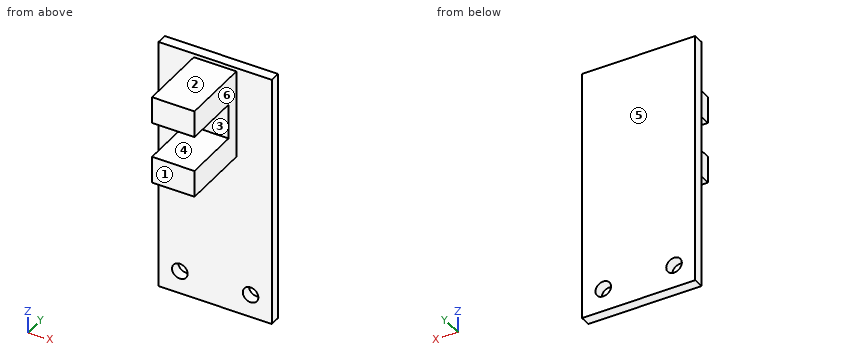
```python
from build123d import *

# Parameters (mm, degrees)
F0_W     = 16
F0_H     = 36
F0_R     = 1.1
F1_DEPTH = 1.47957
F3_W     = 6
F3_H     = 3.8
F4_DEPTH = 10
F3_H_2   = 4.992
F5_DEPTH = 1.85


with BuildPart() as f1:
    # F0 (on Front) → F1 (new body)
    with BuildSketch(Plane.XZ):
        with Locations((8, -18)):
            Rectangle(F0_W, F0_H)
        with Locations((3, -32.75)):
            Circle(F0_R, mode=Mode.SUBTRACT)
        with Locations((13, -32.75)):
            Circle(F0_R, mode=Mode.SUBTRACT)
    extrude(amount=F1_DEPTH)

    # F3 (on face) → F4 (join)
    with BuildSketch(Plane.XZ.offset(1.47957)):
        with Locations((8, -11.192)):
            Rectangle(F3_W, F3_H)
        with Locations((8, -2.4)):
            Rectangle(F3_W, F3_H)
    extrude(amount=F4_DEPTH)

    # F3 (on face) → F5 (join)
    with BuildSketch(Plane.XZ.offset(1.47957)):
        with Locations((8, -6.796)):
            Rectangle(F3_W, F3_H_2)
    extrude(amount=F5_DEPTH)


solid = f1.part
```
Check sheet for the modelled part. Datum: model origin and axes. Units: mm. Face numbers are marked on the shaded views. A direction names the side the tool comes from. Give positions to 0.01 mm unless a question says otherwise; leave off trailing zeros. Order: outer loops, then holes, each group sorted by start corner. A loop starts at its lowest first (then second) coordinate and runs counter-clockwise, first axis right, second up. Notation, with made-up numbers: M 58.25,-4.5 L 87.25,-4.5 A23 ccw 87.25,33.5 Z; hole C 65.25,62.25 d11. An arc over 180 degrees is marked long. Answer in a Markdown table with one row per item. Add a question column.
Q1. Thickness scan on L1, parallel to Z at x = 3, y = -0.55; L2, parallel to Z at x = 10.75, y = -10.5; L3, parallel to Y at x = 9, z = -5. Record the ranges inside material, lowest first.
Q2. Sectioned sample at C-C, the plane z = -32.75. Record the boundary of the cut face in (x, y), and give its area (3 significant figures).
Q3. Sectioned sample at A-A, the plane x = 13. Record the boundary of the cut face in (y, z), and give its area (3 significant figures).
Q4. Sectioned sample at D-D, the plane x = 7. Record the boundary of the cut face in (y, z), and give its area (4 significant figures).
Q5. Gauge pin test, flat ends, axial feed: pin 1 Ø5 at (x, y) = (9, -8) entering from -Z; pin 2 Ø5 at (x, z) = (6, -13.5) entering from -Y; pin 3 Ø2 at (y, z) = (-10, -11.5) entering from -X; pin 4 Ø6.5 at (x, y) = (8.5, -6) entering from +Z. Record the tip position at first contact, or that the pin passes through.
Q6. Access from +Z, -Z, +X, -X, +Y, -Y to the whole of each face (thin tool, end or side, straight path). Record for the marked faces 5 and 6.
Q7. Release check for a two-part mould opening along Z. For the marked faces 1, 2, 3 and 4 record: released by +Z, released by -Z, zero draft, split by the parting line, or undercut.
Q8. Sectioned sample at B-B, the plane y = -5. Record the boundary of the cut face in (x, z), and give its area (3 significant figures).
Verdict:
| question | item | result |
|---|---|---|
| 1 | L1 | -36 to -33.85, -31.65 to 0 |
| 1 | L2 | -13.09 to -9.29, -4.3 to -0.5 |
| 1 | L3 | -3.33 to 0 |
| 2 | outline | M 0,-1.48 L 1.9,-1.48 L 1.9,0 L 0,0 Z; M 4.1,-1.48 L 11.9,-1.48 L 11.9,0 L 4.1,0 Z; M 14.1,-1.48 L 16,-1.48 L 16,0 L 14.1,0 Z |
| 2 | area | 17.2 mm² |
| 3 | outline | M -1.48,-36 L 0,-36 L 0,-33.85 L -1.48,-33.85 Z; M -1.48,-31.65 L 0,-31.65 L 0,0 L -1.48,0 Z |
| 3 | area | 50.0 mm² |
| 4 | outline | M -11.48,-13.09 L -1.48,-13.09 L -1.48,-36 L 0,-36 L 0,0 L -1.48,0 L -1.48,-0.5 L -11.48,-0.5 L -11.48,-4.3 L -3.33,-4.3 L -3.33,-9.29 L -11.48,-9.29 Z |
| 4 | area | 138.5 mm² |
| 5 | pin 1 | z = -13.09 |
| 5 | pin 2 | y = -11.48 |
| 5 | pin 3 | x = 5 |
| 5 | pin 4 | z = -0.5 |
| 6 | face 5 | +Z, -Z, +X, -X, +Y |
| 6 | face 6 | +Z, -Z, +X, -Y |
| 7 | face 1 | zero draft |
| 7 | face 2 | released by +Z |
| 7 | face 3 | undercut |
| 7 | face 4 | undercut |
| 8 | outline | M 5,-13.09 L 11,-13.09 L 11,-9.29 L 5,-9.29 Z; M 5,-4.3 L 11,-4.3 L 11,-0.5 L 5,-0.5 Z |
| 8 | area | 45.6 mm² |
